Model file for the job. Use its own axes, mm. Coordinates: 2 decimals unless noted, no trailing zeros. Write each loop counter-clockwise with the first axis right and the second up, starting at its lowest first coordinate (ties: lowest second). Pieces come first, ordered by that corner, then holes. Notation, with made-up numbers: (14, 3.25) - (37, 3.25) arc R28 cw to (37, 30.25) - close; hole circle Ø7 at (0.25, 68). An arc over 180 degrees is marked (long way). Put each result on its own line as item: value. Start each with the question number.
1. Saw through at C-C, the plane x = 1.8. Write the cut outline in (y, z), plus the area to 3 significant figures.
2. Drill centre lines: L1, parallel to Y at x = 4.05, z = -50; L2, parallel to Z at x = 3.8, y = -1; L3, parallel to Y at x = 1.65, z = 50.5. Where is each one in solid material? Low to high. Write a range as from..to.
3. Saw through at B-B, the plane y = 0. Write the cut outline in (x, z), plus the area to 3 significant figures.
4. Saw through at A-A, the plane z = 50. Write the cut outline in (x, y).
```python
from build123d import *

# Parameters (mm, degrees)
SKETCH_2_W      = 120
SKETCH_2_H      = 10
SKETCH_2_R      = 2
EXTRUDE_1_DEPTH = 5


with BuildPart() as part:
    # 草图2 → 凸台-拉伸1 (new body)
    with BuildSketch(Plane(origin=(0, 0, 0), x_dir=(0, 0, -1), z_dir=(1, 0, 0))):
        Rectangle(SKETCH_2_W, SKETCH_2_H)
        with Locations((-50, 0)):
            Circle(SKETCH_2_R, mode=Mode.SUBTRACT)
        with Locations((50, 0)):
            Circle(SKETCH_2_R, mode=Mode.SUBTRACT)
    extrude(amount=EXTRUDE_1_DEPTH)


solid = part.part
```
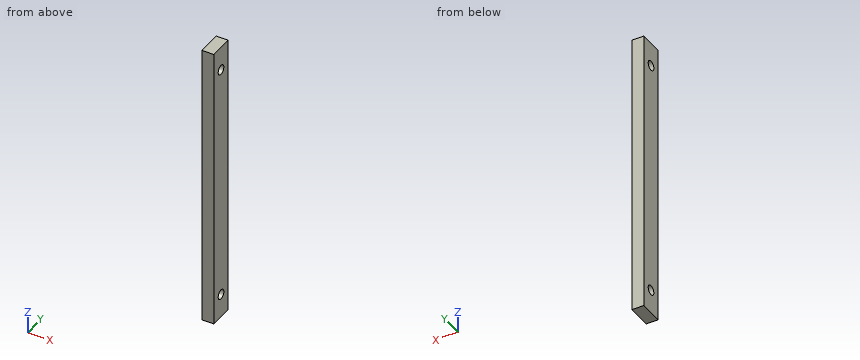
Final values:
1. outline: (-5, -60) - (5, -60) - (5, 60) - (-5, 60) - close; hole circle Ø4 at (0, -50); hole circle Ø4 at (0, 50)
1. area: 1,170 mm²
2. L1: y = -5..-2, 2..5
2. L2: z = -60..-51.73, -48.27..48.27, 51.73..60
2. L3: y = -5..-1.94, 1.94..5
3. outline: (0, -60) - (5, -60) - (5, -52) - (0, -52) - close; (0, -48) - (5, -48) - (5, 48) - (0, 48) - close; (0, 52) - (5, 52) - (5, 60) - (0, 60) - close
3. area: 560 mm²
4. outline: (0, -5) - (5, -5) - (5, -2) - (0, -2) - close; (0, 2) - (5, 2) - (5, 5) - (0, 5) - close
